Geometry: final body of the model. Coordinates: model frame, mm. A direction names the side the tool comes from. Give positions to 0.01 mm unless a question says otherwise; leave off trailing zeros. Write each loop counter-clockwise with the first axis right and the second up, starting at its lowest first coordinate (ties: lowest second). Pieces come first, ordered by that corner, then holes. Notation, with made-up numbers: (82, -24) - (92, -24) arc R15 ccw to (92, 3) - close; hole circle Ø2 at (29, 82). An arc over 180 degrees is marked (long way). Return JSON: item names as keys, results as strings.
from build123d import *

# Parameters (mm, degrees)
SKETCH1_R          = 19.05
EXTRUDE1_DEPTH     = 15.748
SKETCH2_R          = 19.05
SKETCH2_R_2        = 11.049
CUT_EXTRUDE1_DEPTH = 9.398
SKETCH3_R          = 4.7752
CUT_EXTRUDE2_DEPTH = 12.192
CHAMFER1_SIZE      = 0.508


with BuildPart() as part:
    # Sketch1 → Extrude1 (new body)
    with BuildSketch(Plane.XY):
        Circle(SKETCH1_R)
    extrude(amount=EXTRUDE1_DEPTH)

    # Sketch2 → Cut-Extrude1 (cut)
    with BuildSketch(Plane(origin=(0, 0, 0), x_dir=(-1, 0, 0), z_dir=(0, 0, -1))):
        Circle(SKETCH2_R)
        Circle(SKETCH2_R_2, mode=Mode.SUBTRACT)
    extrude(amount=-CUT_EXTRUDE1_DEPTH, mode=Mode.SUBTRACT)

    # Sketch3 → Cut-Extrude2 (cut)
    with BuildSketch(Plane.XY.offset(15.748)):
        Circle(SKETCH3_R)
    extrude(amount=-CUT_EXTRUDE2_DEPTH, mode=Mode.SUBTRACT)

    # Chamfer1
    chamfer1_edges = [part.edges().sort_by_distance(p)[0] for p in [
        (-4.7752, 0, 15.748),
        (11.049, 0, 0),
    ]]
    chamfer(chamfer1_edges, length=CHAMFER1_SIZE)


solid = part.part
Q1. Pin query (flat end, axial travel): P1, Ø5, axis at y = -3.5, z = 11.5, coming from the -X side; P2, Ø1.5, axis at x = 0, y = -11.5, coming from the -Z side; P3, Ø8, axis at x = -7.5, z = 7.5, coming from the +Y side; P4, Ø5, axis at y = 14.5, z = 6, coming from the -X side. Return the tip coordinate at first contact, or that it passes through.
Answer key:
{"P1": "stops at x = -19.02", "P2": "stops at z = 0.21", "P3": "stops at y = 18.63", "P4": "passes through"}
Q2. Section query D-D, the plane z = 1. Return the cut outline in (x, y).
Answer key:
{"outline": "circle Ø22.1 at (0, 0)"}
Q3. Set-up query: faces 4 (the cylindrical face through (-15.12, -11.59, 12.53)), 5 (the flat face through (-8, -8, 9.398)), 6 (the cylindrical face through (-1.04, -4.66, 9.48)). Return all of +Z, -Z, +X, -X, +Y, -Y with unobstructed straight access to the full face (end or side cutting, diameter ignored); none if empty.
Answer key:
{"face 4": "+Z, -Z", "face 5": "-Z", "face 6": "+Z"}
Q4. Section query C-C, the plane z = 5.5. Return the cut outline in (x, y), plus the area to 3 significant figures.
Answer key:
{"outline": "circle Ø22.1 at (0, 0); hole circle Ø9.55 at (0, 0)", "area": "312 mm^2"}
Q5. Material intervals for probe 1 along Y at (x, z) = (0, 10.75); probe 2 along Y at (x, z) = (0, 7.75); probe 3 along Z at (x, y) = (14, 1), sorted ascending. Write a range as [from, to].
Answer key:
{"probe 1": "y = [-19.05, -4.78], [4.78, 19.05]", "probe 2": "y = [-11.05, -4.78], [4.78, 11.05]", "probe 3": "z = [9.4, 15.75]"}
Q6. Mould query, pull axis Y, two halves, no side actions, for faces 1 (the flat face through (0, 0, 3.556)), 2 (the cylindrical face through (1.438, 10.955, 4.891)), 3 (the flat face through (4, -4, 15.748)). Classes: pulls with the +Y half, pulls with the -Y half, needs draft (parallel to the pull), parting line crosses it, or undercut.
Answer key:
{"face 1": "undercut", "face 2": "parting line crosses it", "face 3": "needs draft"}
Q7. Section query A-A, the plane y = 0. Return the cut outline in (x, z), plus the area to 3 significant figures.
Answer key:
{"outline": "(-19.05, 9.4) - (-11.05, 9.4) - (-11.05, 0.51) - (-10.54, 0) - (10.54, 0) - (11.05, 0.51) - (11.05, 9.4) - (19.05, 9.4) - (19.05, 15.75) - (5.28, 15.75) - (4.78, 15.24) - (4.78, 3.56) - (-4.78, 3.56) - (-4.78, 15.24) - (-5.28, 15.75) - (-19.05, 15.75) - close", "area": "333 mm^2"}
